Geometry check sheet. Reference: the model listing, model coordinates, mm. Give positions to 0.01 mm unless a question says otherwise; leave off trailing zeros. Write each loop counter-clockwise with the first axis right and the second up, starting at its lowest first coordinate (ties: lowest second). Pieces come first, ordered by that corner, then holes. Notation, with made-up numbers: (76, 24) - (104, 24) arc R27 ccw to (104, 60) - close; hole circle Ø6 at (-2, 87). An arc over 180 degrees is marked (long way). Write item = value, one per line. Start each with the question number.
(1) Section check C-C, the plane x = 179. Enter the section's corners in (y, z), plus the area to 3 significant figures.
(2) Section check A-A, the plane x = -194. Enter the section's corners in (y, z), plus the area to 4 significant figures.
(3) Thickness scan on L1, parallel to Y at x = -194, z = 7; L2, parallel to Y at x = 165, z = 14; L3, parallel to X at y = 48, z = 5.5. Record the ranges inside material, lowest first.
(4) Section check B-B, the plane z = 3. Enter the section's corners in (x, y), plus the area to 3 significant figures.
(5) Depth check by flat-ended pin: pin 1 Ø2 at (x, z) = (96, 10.5) entering from -Y; pin 2 Ø4 at (y, z) = (40.5, 9) entering from -X; pin 3 Ø1.5 at (y, z) = (40, 9.5) entering from +X. Enter the tip coordinate at first touch or a pass-through.
```python
from build123d import *

# Parameters (mm, degrees)
F0_R     = 10
F1_DEPTH = 15


with BuildPart() as f1:
    # F0 (on Top) → F1 (new body)
    with BuildSketch(Plane.XY):
        Polygon((-360, 32.5), (-360, 0), (360, 0), (360, 32.5), (285, 32.5), (285, 47.5), (360, 47.5), (360, 95), (-360, 95), (-360, 47.5), (-230, 47.5), (-230, 32.5), align=None)
        with Locations((-194, 40)):
            Circle(F0_R, mode=Mode.SUBTRACT)
        with BuildLine():
            ThreePointArc((-119.041678, 42.5), (-117.577212, 46.035534), (-114.041678, 47.5))
            Line((-114.041678, 47.5), (195.958322, 47.5))
            ThreePointArc((195.958322, 47.5), (199.493856, 46.035534), (200.958322, 42.5))
            Line((200.958322, 42.5), (200.958322, 37.5))
            ThreePointArc((200.958322, 37.5), (199.493856, 33.964466), (195.958322, 32.5))
            Line((195.958322, 32.5), (-114.041678, 32.5))
            ThreePointArc((-114.041678, 32.5), (-117.577212, 33.964466), (-119.041678, 37.5))
            Line((-119.041678, 37.5), (-119.041678, 42.5))
        make_face(mode=Mode.SUBTRACT)
    extrude(amount=F1_DEPTH)


solid = f1.part
```
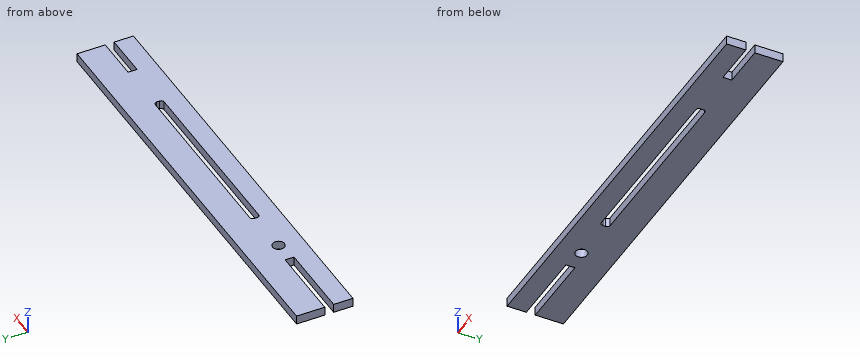
Model answer:
q1.outline = (0, 0) - (32.5, 0) - (32.5, 15) - (0, 15) - close; (47.5, 0) - (95, 0) - (95, 15) - (47.5, 15) - close
q1.area = 1,200 mm²
q2.outline = (0, 0) - (30, 0) - (30, 15) - (0, 15) - close; (50, 0) - (95, 0) - (95, 15) - (50, 15) - close
q2.area = 1,125 mm²
q3.L1 = 0 to 30, 50 to 95
q3.L2 = 0 to 32.5, 47.5 to 95
q3.L3 = -360 to -200, -188 to 360
q4.outline = (-360, 0) - (360, 0) - (360, 32.5) - (285, 32.5) - (285, 47.5) - (360, 47.5) - (360, 95) - (-360, 95) - (-360, 47.5) - (-230, 47.5) - (-230, 32.5) - (-360, 32.5) - close; hole circle Ø20 at (-194, 40); hole (-119.04, 37.5) arc R5 ccw to (-114.04, 32.5) - (195.96, 32.5) arc R5 ccw to (200.96, 37.5) - (200.96, 42.5) arc R5 ccw to (195.96, 47.5) - (-114.04, 47.5) arc R5 ccw to (-119.04, 42.5) - close
q4.area = 60,200 mm²
q5.pin_1 = 0
q5.pin_2 = -230
q5.pin_3 = 285
